Autodesk Inventor part; units mm, degrees
ref_plane "YZ Plane" through (0, 0, 0) normal (1, 0, 0) x (0, 1, 0)
ref_plane "XZ Plane" through (0, 0, 0) normal (0, 1, 0) x (-1, 0, 0)
ref_plane "XY Plane" through (0, 0, 0) normal (0, 0, 1) x (1, 0, 0)
sketch "Sketch1" plane through (0, 0, 0) normal (0, 1, 0) x (-1, 0, 0)
  line L0 (162.815, -12.8435) -> (-162.815, -12.8435)
  line L1 (-162.815, -12.8435) -> (-162.815, 12.8435)
  line L2 (-162.815, 12.8435) -> (162.815, 12.8435)
  line L3 (162.815, 12.8435) -> (162.815, -12.8435)
  point P0 (0, 0)
  point P1 (162.815, 0)
  point P2 (0, -12.8435)
  dimension "d0" = 325.63
  dimension "d2" = 25.687
extrude "Extrusion1" add sketch "Sketch1" along normal blind 12.7
draft "FaceDraft1" angle -10 pull direction (0, -1, 0) faces at (162.815, 8.4667, -4.2812) fixed edges at (162.815, 0, 0)
draft "FaceDraft2" angle -10 pull direction (0, -1, 0) faces at (-162.815, 8.4667, 4.2812) fixed edges at (-162.815, 0, 0)
draft "FaceDraft3" angle 10 pull direction (0, -1, 0) faces at (53.5252, 4.2333, 12.8435) fixed edges at (0, 0, 12.8435)
properties part number "Panel_front"
Here's how the part is built. I have some questions about the finished solid (model axes, mm). Coordinates: 2 decimals unless noted, no trailing zeros. Loops run counter-clockwise (first coordinate to the right, second up) from the corner with the lowest first, then second, coordinate; pieces in that order, holes last. Notation, with made-up numbers: (75.25, 80) -> (119.25, 80) arc R30 ccw to (119.25, 107) -> close; hole circle Ø6 at (70.25, -25.5). An arc over 180 degrees is marked (long way). Return JSON: item names as keys, results as strings.
1) Will these pins go through, and if not, where does the flat tip stop? pin 1 (2 mm diameter, centred on y = 10, z = -2, fed in from -X); pin 2 (1.5 mm diameter, centred on y = 11, z = 2.5, fed in from -X); pin 3 (1.5 mm diameter, centred on y = 2, z = -7.5, fed in from +X).
Results below:
{"pin 1": "x = -161.23", "pin 2": "x = -161.01", "pin 3": "x = 162.59"}
2) If we section it at A-A, the plane x = 58: Write out the boundary of the cut face in (y, z), then the cut area to 3 significant figures.
Results below:
{"outline": "(0, -12.84) -> (12.7, -12.84) -> (12.7, 15.08) -> (0, 12.84) -> close", "area": "340 mm²"}
3) I need wall thicknesses on line 1 (Z direction, x = 127, y = 5.25); line 2 (X direction, y = 11.25, z = -0.75); line 3 (Z direction, x = 123, y = 3.75). Which ranges of each line are inside material? Lowest first, please. Write a range as from..to.
Results below:
{"line 1": "-12.84..13.77", "line 2": "-160.83..160.83", "line 3": "-12.84..13.5"}
4) If we section it at B-B, the plane y = 6.25: Write out the boundary of the cut face in (x, z).
Results below:
{"outline": "(-161.71, -12.84) -> (161.71, -12.84) -> (161.71, 13.95) -> (-161.71, 13.95) -> close"}
